The listing builds one solid part. Answer for the finished solid, in the listing's coordinates (mm). A direction names the side the tool comes from. Give positions to 0.01 mm unless a question says otherwise; leave off trailing zeros. Order: outer loops, then holes, each group sorted by start corner. A loop starts at its lowest first (then second) coordinate and runs counter-clockwise, first axis right, second up. Notation, with made-up numbers: (-1.5, -38.75) - (30.5, -38.75) arc R7 ccw to (30.5, -27.75) - close; hole circle Ø4 at (-32, 52). An arc over 180 degrees is marked (long way). Answer as CSV lines item,"result". Start each with the question number.
1. Consider line 1 along Z through (x, y) = (-9, 5.5); line 2 along Y through (x, z) = (2.5, 4.55); line 3 along Y through (x, z) = (-1.75, 4.25). Determine where each line is inside the solid, lowest interval first. Write a range as [from, to].
2. Section D-D on y = -3.5 is taken. Give the vertices of the cut face in (x, z).
3. Section A-A on z = 5.4 is taken. Count the separate pieces of the cut face and the enclosed holes in it, and give its area (3 significant figures).
4. Section B-B on z = 2.05 is taken. Give the vertices of the cut face in (x, y), and give its area (3 significant figures).
5. Flat-ended cylindrical pins translate along their axes: pin 1 (2 mm diameter, centred on x = 4.5, z = 2, fed in from +Y); pin 2 (1.5 mm diameter, centred on x = 0, z = 5, fed in from -Y); pin 3 (1 mm diameter, centred on x = -10, z = 1.5, fed in from +Y). Find the tip coordinate at first contact, or state that the pin passes through.
6. Which of the six approach directions +Z, -Z, +X, -X, +Y, -Y give full straight-line access (tool end or side, diameter ignored) to faces 5 (the flat face through (-11.769, -0.924, 4.479)), 6 (the flat face through (4.04, -11.13, 4.48)), 7 (the flat face through (7.635, 1.681, 4.479))?
7. Section C-C on y = -9 is taken. Give the vertices of the cut face in (x, z), and give its area (3 significant figures).
8. Determine the mould class of faces 1 (the flat face through (0, 10.5, 4)), 2 (the flat face through (-8.45, -8.3, 4.48)), 3 (the flat face through (-7, 2, 6)), 4 (the flat face through (-0.74, 11.82, 4.48)) for opening direction Y: +Y half, -Y half, draft (parallel to the pull), parting line (faces both ways), or undercut.
from build123d import *

# Parameters (mm, degrees)
F0_R     = 14
F1_DEPTH = 3
F3_DEPTH = 3


# Not quite as in the source:
# - a feature names something its author has since deleted; it is built from what else it names


with BuildPart() as f1:
    # F0 (on Top) → F1 (new body)
    with BuildSketch(Plane.XY):
        Circle(F0_R)
    extrude(amount=F1_DEPTH)

    # F2 (on face) → F3 (join)
    with BuildSketch(Plane.XY.offset(3)):
        Polygon((0, 6.5), (1.5, 6.5), (0, 9.0980762114), (-1.5, 6.5), align=None)
        Polygon((-6.6453928475, 0.582025689), (-6.1818673809, 2.0086103865), (-5.7183418644, 3.4351952379), (-8.6527846666, 2.8114601654), align=None)
        Polygon((-2.6070786483, -6.1402883419), (-3.8206041381, -5.2586104647), (-5.0341296315, -4.376932585), (-5.3477150213, -7.3604982711), align=None)
        Polygon((-6.9386088825, 8.0222008685), (-5.6767273349, 8.833162897), (-4.414848284, 9.6441233209), (-7.08135463, 11.0188028861), align=None)
        Polygon((0, 10.5), (1.5, 10.5), (0, 13.0980762114), (-1.5, 10.5), align=None)
        Polygon((4.3974313073, -9.6520773877), (2.9581918265, -10.0746762289), (1.5189523864, -10.4972750582), (3.6901545007, -12.5675120927), align=None)
        Polygon((-1.5189523864, -10.4972750582), (-2.9581918467, -10.074676223), (-4.3974313073, -9.6520773877), (-3.6901545007, -12.5675120927), align=None)
        Polygon((-6.9530794298, -8.009662068), (-7.9353704205, -6.8760378337), (-8.9176616316, -5.7424133449), (-9.8988655216, -8.577415801), align=None)
        Polygon((-10.1796528823, -2.9790379647), (-10.3931251437, -1.4943057747), (-10.6065973972, -0.009573639), (-12.9647566814, -1.8640505977), align=None)
        Polygon((0, 2.5), (1.5, 2.5), (0, 5.0980762114), (-1.5, 2.5), align=None)
        Polygon((-1.4150635095, -2.5490381057), (-2.1650632679, -1.2500004183), (-2.9150635095, 0.0490381057), (-4.4150635095, -2.5490381057), align=None)
        Polygon((2.9150635095, 0.0490381057), (2.1650632692, -1.2500004162), (1.4150635095, -2.5490381057), (4.4150635095, -2.5490381057), align=None)
        Polygon((8.9280134317, 5.7263056296), (9.5511359728, 4.3618575893), (10.1742584707, 2.9974096435), (11.9144291994, 5.4411374996), align=None)
        Polygon((5.7183418644, 3.4351952379), (6.1818673459, 2.0086104943), (6.6453928475, 0.582025689), (8.6527846666, 2.8114601654), align=None)
        Polygon((5.0341296315, -4.376932585), (3.8206041381, -5.2586104647), (2.6070786483, -6.1402883419), (5.3477150213, -7.3604982711), align=None)
        Polygon((8.9176616316, -5.7424133449), (7.9353705512, -6.8760376828), (6.9530794298, -8.009662068), (9.8988655216, -8.577415801), align=None)
        Polygon((10.6065973972, -0.009573639), (10.3931251437, -1.4943057747), (10.1796528823, -2.9790379647), (12.9647566814, -1.8640505977), align=None)
        Polygon((-10.1742584707, 2.9974096435), (-9.551135936, 4.3618576698), (-8.9280134317, 5.7263056296), (-11.9144291994, 5.4411374996), align=None)
        Polygon((4.414848284, 9.6441233209), (5.6767273496, 8.8331628876), (6.9386088825, 8.0222008685), (7.08135463, 11.0188028861), align=None)
    extrude(amount=F3_DEPTH)


solid = f1.part
Checks:
1,line 1,"z = [0, 3]"
1,line 2,"y = [-11.43, -10.21], [-2.55, -0.67]"
1,line 3,"y = [-10.72, -10.43], [-2.55, -1.97]"
2,outline,"(-13.56, 0) - (13.56, 0) - (13.56, 3) - (-13.56, 3) - close"
3,separate pieces,"19"
3,enclosed holes,"0"
3,area,"74.0 mm²"
4,outline,"circle Ø28 at (0, 0)"
4,area,"616 mm²"
5,pin 1,"stops at y = 13.56"
5,pin 2,"stops at y = 2.5"
5,pin 3,"stops at y = 10.28"
6,face 5,"+Z, -X"
6,face 6,"+Z, +X, -Y"
6,face 7,"+Z, +X"
7,outline,"(-10.72, 0) - (10.72, 0) - (10.72, 3) - (-10.72, 3) - close"
7,area,"64.3 mm²"
8,face 1,"undercut"
8,face 2,"-Y half"
8,face 3,"draft"
8,face 4,"+Y half"
